Work out the finished part from the listing and answer in its coordinate system (mm). Round coordinates to 2 decimals unless told otherwise and drop trailing zeros. Order: outer loops, then holes, each group sorted by start corner. A loop starts at its lowest first (then second) coordinate and runs counter-clockwise, first axis right, second up. Notation, with made-up numbers: (43.25, -26.5) - (86.25, -26.5) arc R16 ccw to (86.25, 1.5) - close; hole circle Ø9 at (-2, 4). An arc over 180 degrees is marked (long way). Answer in a Markdown table with one row per item.
from build123d import *

# Parameters (mm, degrees)
BOSS_EXTRU_1_DEPTH      = 2
ESQUISSE2_R             = 1.6
ENL_V_MAT_EXTRU_1_DEPTH = 10


with BuildPart() as part:
    # Esquisse1 → Boss.-Extru.1 (new body)
    with BuildSketch(Plane.XY):
        Polygon((80, 160), (40, 160), (40, 42), (54, 42), (54, 0), (80, 0), align=None)
        Polygon((40, 42), (40, 160), (0, 160), (0, 0), (26, 0), (26, 42), align=None)
    extrude(amount=BOSS_EXTRU_1_DEPTH)

    # Esquisse2 → Enlèv. mat.-Extru.1 (cut)
    with BuildSketch(Plane.XY):
        with Locations((5, 145)):
            Circle(ESQUISSE2_R)
        with Locations((5, 5)):
            Circle(ESQUISSE2_R)
        with Locations(Location((75, 5, 0), (0, 0, 180))):
            Circle(ESQUISSE2_R)
        with Locations(Location((75, 145, 0), (0, 0, 180))):
            Circle(ESQUISSE2_R)
    extrude(amount=ENL_V_MAT_EXTRU_1_DEPTH, mode=Mode.SUBTRACT)


solid = part.part
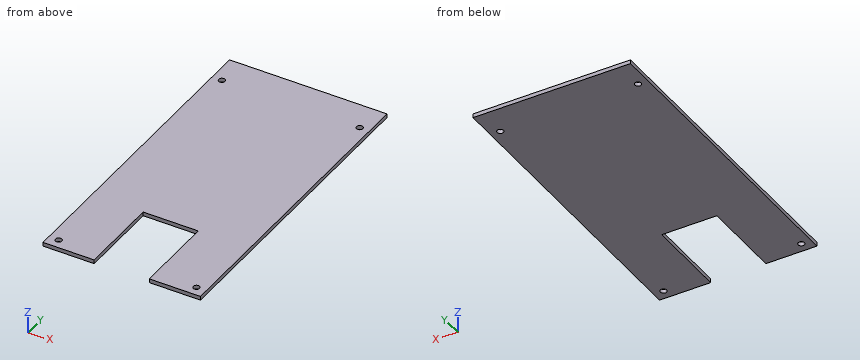
1) This flat-tipped pin is pushed along its axis until it touches: pin 1 (1 mm diameter, centred on x = 60, y = 114.5, fed in from -Z). Where does it stop, or does it pass through?
Filled in:
| item | result |
|---|---|
| pin 1 | stops at z = 0 |
2) Find section B-B, the plane x = 5. Give the vertices of the cut face in (y, z).
Filled in:
| item | result |
|---|---|
| outline | (0, 0) - (3.4, 0) - (3.4, 2) - (0, 2) - close; (6.6, 0) - (143.4, 0) - (143.4, 2) - (6.6, 2) - close; (146.6, 0) - (160, 0) - (160, 2) - (146.6, 2) - close |
3) Find section C-C, the plane y = 145. Give the vertices of the cut face in (x, z).
Filled in:
| item | result |
|---|---|
| outline | (0, 0) - (3.4, 0) - (3.4, 2) - (0, 2) - close; (6.6, 0) - (73.4, 0) - (73.4, 2) - (6.6, 2) - close; (76.6, 0) - (80, 0) - (80, 2) - (76.6, 2) - close |
4) Find section D-D, the plane y = 5. Give the vertices of the cut face in (x, z).
Filled in:
| item | result |
|---|---|
| outline | (0, 0) - (3.4, 0) - (3.4, 2) - (0, 2) - close; (6.6, 0) - (26, 0) - (26, 2) - (6.6, 2) - close; (54, 0) - (73.4, 0) - (73.4, 2) - (54, 2) - close; (76.6, 0) - (80, 0) - (80, 2) - (76.6, 2) - close |
5) Find the intervals of material crossed by probe 1 along Y at (x, z) = (75, 0.8); probe 2 along X at (y, z) = (145, 1.1); probe 3 along X at (y, z) = (5, 1), in increasing order. Write a range as from..to.
Filled in:
| item | result |
|---|---|
| probe 1 | y = 0..3.4, 6.6..143.4, 146.6..160 |
| probe 2 | x = 0..3.4, 6.6..73.4, 76.6..80 |
| probe 3 | x = 0..3.4, 6.6..26, 54..73.4, 76.6..80 |
6) Find section A-A, the plane y = 33.5. Give the vertices of the cut face in (x, z).
Filled in:
| item | result |
|---|---|
| outline | (0, 0) - (26, 0) - (26, 2) - (0, 2) - close; (54, 0) - (80, 0) - (80, 2) - (54, 2) - close |
